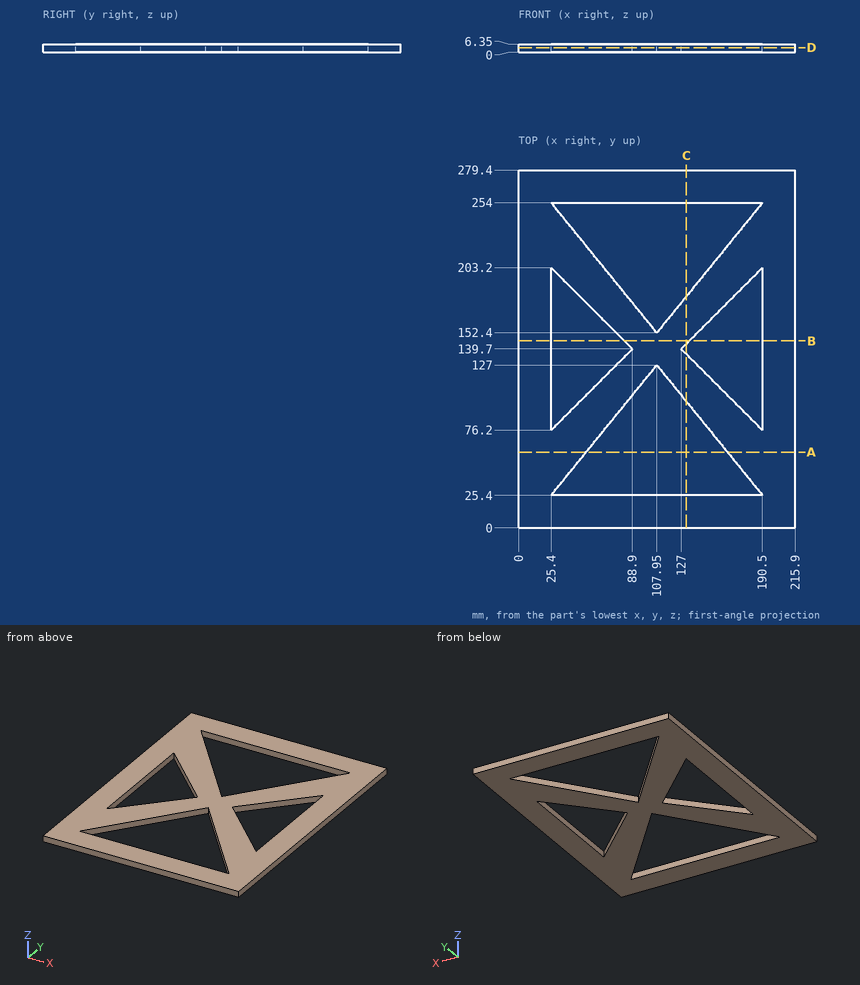
The drawing under review shows one solid part. Ordinate dimensions are in mm from its lowest x, y, z. Coordinates: 2 decimals unless noted, no trailing zeros. Write each loop counter-clockwise with the first axis right and the second up, starting at its lowest first coordinate (ties: lowest second). Pieces come first, ordered by that corner, then holes.
1) To check wall thickness, follow L1, parallel to Y at x = 97, z = 3.75; L2, parallel to X at y = 82.5, z = 1.5; L3, parallel to X at y = 126.5, z = 0.5. State the ranges of each line that lie inside material, in increasing order.
2) Add section B-B (y = 146). Write out the cut boundary in (x, z).
3) Add section A-A (y = 59). Write out the cut boundary in (x, z), plus the area to 3 significant figures.
4) Add section D-D (z = 3.5). Write out the cut boundary in (x, y).
5) Add section C-C (x = 131). Write out the cut boundary in (y, z).
Check result:
1. L1: y = 0 to 25.4, 113.52 to 165.88, 254 to 279.4
1. L2: x = 0 to 25.4, 31.7 to 71.79, 144.11 to 184.2, 190.5 to 215.9
1. L3: x = 0 to 25.4, 75.7 to 107.54, 108.36 to 140.2, 190.5 to 215.9
2. outline: (0, 0) - (25.4, 0) - (25.4, 6.35) - (0, 6.35) - close; (82.6, 0) - (133.3, 0) - (133.3, 6.35) - (82.6, 6.35) - close; (190.5, 0) - (215.9, 0) - (215.9, 6.35) - (190.5, 6.35) - close
3. outline: (0, 0) - (52.7, 0) - (52.7, 6.35) - (0, 6.35) - close; (163.2, 0) - (215.9, 0) - (215.9, 6.35) - (163.2, 6.35) - close
3. area: 669 mm2
4. outline: (0, 0) - (215.9, 0) - (215.9, 279.4) - (0, 279.4) - close; hole (25.4, 25.4) - (190.5, 25.4) - (107.95, 127) - close; hole (25.4, 76.2) - (88.9, 139.7) - (25.4, 203.2) - close; hole (25.4, 254) - (107.95, 152.4) - (190.5, 254) - close; hole (127, 139.7) - (190.5, 76.2) - (190.5, 203.2) - close
5. outline: (0, 0) - (25.4, 0) - (25.4, 6.35) - (0, 6.35) - close; (98.63, 0) - (135.7, 0) - (135.7, 6.35) - (98.63, 6.35) - close; (143.7, 0) - (180.77, 0) - (180.77, 6.35) - (143.7, 6.35) - close; (254, 0) - (279.4, 0) - (279.4, 6.35) - (254, 6.35) - close
